The listing builds one solid part. Answer for the finished solid, in the listing's coordinates (mm). Give positions to 0.01 mm unless a question says otherwise; leave off trailing zeros. Loops run counter-clockwise (first coordinate to the right, second up) from the corner with the lowest first, then second, coordinate; pieces in that order, holes last. Notation, with made-up numbers: M 36,48.5 L 56,48.5 A19 ccw 56,63.5 Z; hole C 53.25,-22.75 d11. An arc over 180 degrees is marked long. One line per item, written item: value. Start each with the question number.
Q1. Consider L1, parallel to Z at x = 3, y = -0.4; L2, parallel to Z at x = -5.5, y = -0.4; L3, parallel to X at y = -0.4, z = 39. Determine where each line is inside the solid, lowest interval first.
Q2. A cutting plane is placed at B-B, the plane x = 0. Determine the outline of the cut face in (y, z), and give its area (3 significant figures).
Q3. A cutting plane is placed at C-C, the plane y = -1.3. Determine the outline of the cut face in (x, z), and give its area (3 significant figures).
Q4. A cutting plane is placed at D-D, the plane z = 34. Determine the outline of the cut face in (x, y), and give its area (3 significant figures).
Q5. A cutting plane is placed at A-A, the plane z = -21. Determine the outline of the cut face in (x, y).
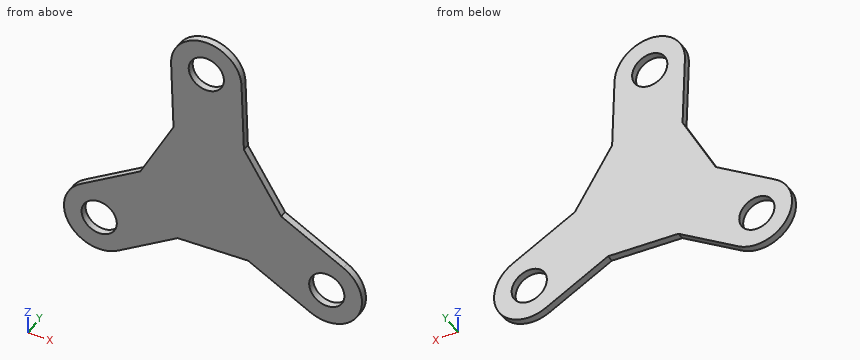
from build123d import *

# Parameters (mm, degrees)
BASE_FLANGE1_DEPTH = 2
SKETCH9_R          = 5
TAB1_DEPTH         = 2


# Sheet-metal steps are written as plain solids
with BuildPart() as part:
    # Sketch1 → Base-Flange1 (new body)
    with BuildSketch(Plane(origin=(0, 0, 0), x_dir=(1, 0, 0), z_dir=(0, 1, 0))):
        Polygon((10.580822677, 16.971923623), (-9.40770567, 17.649223043), (-19.988528347, 0.67729942), (-10.580822677, -16.971923623), (9.40770567, -17.649223043), (19.988528347, -0.67729942), align=None)
    extrude(amount=-BASE_FLANGE1_DEPTH)

    # Sketch9 → Tab1 (add)
    # profile 1 of 3: a face of its own
    with BuildSketch(Plane.XZ.offset(2)):
        with BuildLine():
            Line((-10.580822677, 16.971923623), (-11.258122097, 36.960451971))
            ThreePointArc((-11.258122097, 36.960451971), (-1.602507633, 47.293365854), (8.73040625, 37.63775139))
            Line((8.73040625, 37.63775139), (9.40770567, 17.649223043))
            Line((9.40770567, 17.649223043), (-10.580822677, 16.971923623))
        make_face()
        with Locations(Location((-1.263857923, 37.299101681, 0), (0, 0, 270))):
            Circle(SKETCH9_R, mode=Mode.SUBTRACT)
    # profile 2 of 3: a face of its own
    with BuildSketch(Plane.XZ.offset(2)):
        with BuildLine():
            Line((19.988528347, 0.67729942), (37.63775139, -8.73040625))
            ThreePointArc((37.63775139, -8.73040625), (41.758510077, -22.258870607), (28.23004572, -26.379629293))
            Line((28.23004572, -26.379629293), (10.580822677, -16.971923623))
            Line((10.580822677, -16.971923623), (19.988528347, 0.67729942))
        make_face()
        with Locations(Location((32.933898555, -17.555017772, 0), (0, 0, 270))):
            Circle(SKETCH9_R, mode=Mode.SUBTRACT)
    # profile 3 of 3: a face of its own
    with BuildSketch(Plane.XZ.offset(2)):
        with BuildLine():
            Line((-9.40770567, -17.649223043), (-26.379629293, -28.23004572))
            ThreePointArc((-26.379629293, -28.23004572), (-40.156002444, -25.034495247), (-36.960451971, -11.258122097))
            Line((-36.960451971, -11.258122097), (-19.988528347, -0.67729942))
            Line((-19.988528347, -0.67729942), (-9.40770567, -17.649223043))
        make_face()
        with Locations(Location((-31.670040632, -19.744083909, 0), (0, 0, 270))):
            Circle(SKETCH9_R, mode=Mode.SUBTRACT)
    extrude(amount=-TAB1_DEPTH)


solid = part.part
Answer block:
1. L1: -17.23 to 34.69, 39.91 to 46.34
1. L2: -17.52 to 34.64, 39.96 to 46.36
1. L3: -11.12 to -5.97, 3.44 to 8.59
2. outline: M -2,-17.33 L 0,-17.33 L 0,32.46 L -2,32.46 Z; M -2,42.14 L 0,42.14 L 0,47.22 L -2,47.22 Z
2. area: 110 mm^2
3. outline: M -36.96,-11.26 A10 ccw -26.38,-28.23 L -9.41,-17.65 L 10.58,-16.97 L 28.23,-26.38 A10 ccw 37.64,-8.73 L 19.99,0.68 L 9.41,17.65 L 8.73,37.64 A10 ccw -11.26,36.96 L -10.58,16.97 L -19.99,-0.68 Z; hole C -31.67,-19.74 d10; hole C -1.26,37.3 d10; hole C 32.93,-17.56 d10
3. area: 2,470 mm^2
4. outline: M -11.16,-2 L -5.02,-2 L -5.02,0 L -11.16,0 Z; M 2.49,-2 L 8.85,-2 L 8.85,0 L 2.49,0 Z
4. area: 25.0 mm^2
5. outline: M -41.59,-2 L -36.51,-2 L -36.51,0 L -41.59,0 Z; M -26.83,-2 L -14.78,-2 L -14.78,0 L -26.83,0 Z; M 18.14,-2 L 29.31,-2 L 29.31,0 L 18.14,0 Z; M 36.56,-2 L 42.32,-2 L 42.32,0 L 36.56,0 Z
